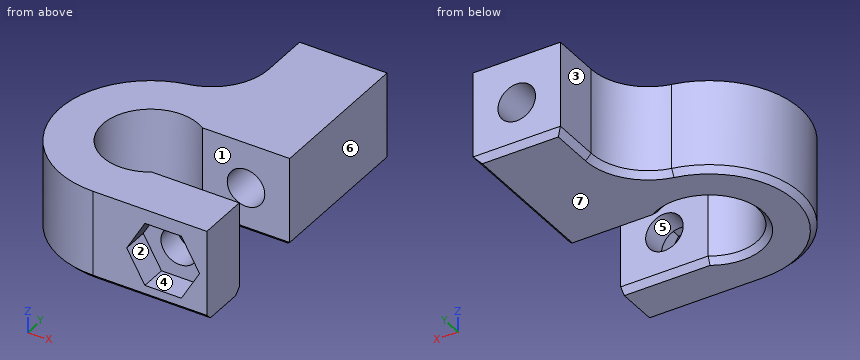
from build123d import *

# Parameters (mm, degrees)
BOSS_EXTRUDE1_DEPTH = 8
SKETCH2_R           = 1.65
CUT_EXTRUDE1_DEPTH  = 21.493901532
CUT_EXTRUDE2_DEPTH  = 2.3
SKETCH4_W           = 7.678362647
SKETCH4_H           = 8
SKETCH4_R           = 1.65
BOSS_EXTRUDE2_DEPTH = 13.5
FILLET1_R           = 5
CHAMFER1_SIZE       = 0.5


with BuildPart() as part:
    # Sketch1 → Boss-Extrude1 (new body)
    with BuildSketch(Plane.XY):
        with BuildLine():
            Line((0, 8), (10, 8))
            Line((10, 8), (10, 3.5))
            Line((10, 3.5), (2.321637353, 3.5))
            ThreePointArc((2.321637353, 3.5), (-4.2, 0), (2.321637353, -3.5))
            Line((2.321637353, -3.5), (10, -3.5))
            Line((10, -3.5), (10, -8))
            Line((10, -8), (0, -8))
            ThreePointArc((0, -8), (-8, 0), (0, 8))
        make_face()
    extrude(amount=BOSS_EXTRUDE1_DEPTH)

    # Sketch2 → Cut-Extrude1 (cut, through all)
    with BuildSketch(Plane.XZ.offset(8)):
        with Locations(Location((6.16, 4, 0), (0, 0, 270))):
            Circle(SKETCH2_R)
    extrude(amount=-CUT_EXTRUDE1_DEPTH, mode=Mode.SUBTRACT)

    # Sketch3 → Cut-Extrude2 (cut)
    with BuildSketch(Plane.XZ.offset(8)):
        Polygon((7.76, 6.771281292), (4.56, 6.771281292), (2.96, 4), (4.56, 1.228718708), (7.76, 1.228718708), (9.36, 4), align=None)
    extrude(amount=-CUT_EXTRUDE2_DEPTH, mode=Mode.SUBTRACT)

    # Sketch4 → Boss-Extrude2 (add)
    with BuildSketch(Plane.XZ.offset(-3.5)):
        with Locations((6.160818676, 4)):
            Rectangle(SKETCH4_W, SKETCH4_H)
        with Locations(Location((6.16, 4, 0), (0, 0, 270))):
            Circle(SKETCH4_R, mode=Mode.SUBTRACT)
    extrude(amount=-BOSS_EXTRUDE2_DEPTH)

    # Fillet1
    fillet1_edges = [part.edges().sort_by_distance(p)[0] for p in [
        (2.321637353, 8, 4),
    ]]
    fillet(fillet1_edges, radius=FILLET1_R)

    # Chamfer1
    chamfer1_edges = [part.edges().sort_by_distance(p)[0] for p in [
        (5, -8, 0),
        (-7.956976548, -0.828567563, 0),
        (1.204335989, 9.570758083, 0),
        (2.321637353, 14.860549771, 0),
        (6.160818677, 17, 0),
        (10, 10.25, 0),
        (6.160818677, 3.5, 0),
        (6.160818677, -3.5, 0),
        (-4.2, 0, 0),
    ]]
    chamfer(chamfer1_edges, length=CHAMFER1_SIZE)


solid = part.part
Geometry: final body of the model. Coordinates: model frame, mm. Face numbers are marked on the shaded views. A direction names the side the tool comes from. Round coordinates to 2 decimals unless told otherwise and drop trailing zeros. Loops run counter-clockwise (first coordinate to the right, second up) from the corner with the lowest first, then second, coordinate; pieces in that order, holes last.
Q1. Material intervals for L1, parallel to Y at x = 5.5, z = 7.25; L2, parallel to Y at x = 7, z = 6.25; L3, parallel to X at y = -4.95, z = 4, sorted ascending.
Q2. Pin query (flat end, axial travel): P1, Ø3, axis at x = 6, z = 5, coming from the -Y side; P2, Ø2, axis at y = 15.5, z = 3.5, coming from the -X side; P3, Ø3, axis at y = 1.5, z = 4.5, coming from the -X side; P4, Ø5, axis at x = 0, y = 0, coming from the +Z side. Return the tip coordinate at first contact, or that it passes through.
Q3. Pull-direction query (X, two-part tool) for the marked faces 4, 5, 6 and 7; classes: released by +X, released by -X, zero draft, split by the parting line, or undercut.
Q4. Access query for the marked faces 1, 2 and 3. Directions: +Z, -Z, +X, -X, +Y, -Y. A direction counts if a zero-diameter tool reaches every point of the face in a straight line with its end or side. Return the directions, or none.
Q5. Section C-C on y = 0. Return loops of the section in (x, z), plus the area to 4 significant figures.
Q6. Section B-B on x = 8.5. Return loops of the section in (y, z), plus the area to 3 significant figures.
Q7. Section A-A on x = 6.16. Return loops of the section in (y, z), plus the area to 3 significant figures.
Evaluation:
1. L1: y = -8 to -3.5, 3.5 to 17
1. L2: y = -5.7 to -3.5, 3.5 to 17
1. L3: x = -6.28 to 4.51, 7.81 to 10
2. P1: stops at y = -5.7
2. P2: stops at x = 2.32
2. P3: stops at x = -8
2. P4: passes through
3. face 4: undercut
3. face 5: undercut
3. face 6: released by +X
3. face 7: zero draft
4. face 1: +Z, -Z, +X
4. face 2: -Y
4. face 3: +Z, -Z, -X, +Y
5. outline: (-8, 0.5) - (-7.5, 0) - (-4.7, 0) - (-4.2, 0.5) - (-4.2, 8) - (-8, 8) - close
5. area: 30.15 mm2
6. outline: (-8, 0.5) - (-7.5, 0) - (-4, 0) - (-3.5, 0.5) - (-3.5, 8) - (-8, 8) - (-8, 5.49) - (-5.7, 5.49) - (-5.7, 2.51) - (-8, 2.51) - close; (3.5, 0.5) - (4, 0) - (16.5, 0) - (17, 0.5) - (17, 8) - (3.5, 8) - close
6. area: 137 mm2
7. outline: (-8, 0.5) - (-7.5, 0) - (-4, 0) - (-3.5, 0.5) - (-3.5, 2.35) - (-5.7, 2.35) - (-5.7, 1.23) - (-8, 1.23) - close; (-8, 6.77) - (-5.7, 6.77) - (-5.7, 5.65) - (-3.5, 5.65) - (-3.5, 8) - (-8, 8) - close; (3.5, 0.5) - (4, 0) - (16.5, 0) - (17, 0.5) - (17, 2.35) - (3.5, 2.35) - close; (3.5, 5.65) - (17, 5.65) - (17, 8) - (3.5, 8) - close
7. area: 78.9 mm2
